For this review, take the finished solid that the model builds, in its own axes (mm). A direction names the side the tool comes from. Coordinates: 2 decimals unless noted, no trailing zeros. Loops run counter-clockwise (first coordinate to the right, second up) from the corner with the lowest first, then second, coordinate; pieces in that order, holes last. Notation, with made-up numbers: (46.25, -16) - (82.25, -16) arc R17 cw to (82.25, 2) - close; hole circle Ø7 at (66, -21). An arc over 180 degrees is marked (long way). Answer as a JSON object with one key per item and string values. Group by question number.
Item 1: Tool access review of faces 1 (the flat face through (-1.727, -0.979, 9.569)), 2 (the flat face through (0, 0, 0)): name each direction out of +Z, -Z, +X, -X, +Y, -Y from which nothing blocks a thin tool from reaching the whole face with its end or side.
Item 2: To check wall thickness, follow line 1 (Y direction, x = 0, z = 11) (3 decimals); line 2 (Z direction, x = 0.5, y = -1); line 3 (X direction, y = -2.25, z = 6.25). State the ranges of each line that lie inside material, in increasing order.
Item 3: Clearance check with flat-ended pins moving along their axes: pin 1 (2 mm diameter, centred on x = -2.5, z = 10.5, fed in from -Y); pin 2 (1.5 mm diameter, centred on y = 2.5, z = 6, fed in from +X). State where each tip first meets the part, or that it passes through.
Item 4: Mouldability with a two-part tool opening along Y and no side actions: class faces 3 (the flat face through (-1.71, 1.01, 9.57)), 4 (the cylindrical face through (3.666, 1.52, 6.269)), 5 (the flat face through (1.71, -1.01, 9.57)), 6 (the flat face through (-2, -1, 12.7)) as released by +Y, released by -Y, zero draft, split by the parting line, or undercut.
Item 5: We need section A-A (z = 8.75). Give the boundary of the cut face in (x, y) (3 decimals).
Item 6: We need section C-C (z = 3.25). Give the boundary of the cut face in (x, y).
Solid Edge part; units mm, degrees
sketch "Sketch1" plane through (0, 0, 0) normal (0, 0, 1) x (1, 0, 0)
  circle A0 centre (0, 0) radius 3.9688
extrude "Protrusion1" add sketch "Sketch1" along normal blind 12.7
chamfer "Chamfer1" distance 0.5953 angle 45 2 edges at (-3.9687, 0, 0) (-3.9687, 0, 12.7)
sketch "Sketch2" plane through (0, 0, 12.7) normal (0, 0, 1) x (1, 0, 0)
  line L0 (-1.146, 1.985) -> (1.146, 1.985)
  line L1 (2.2921, 0) -> (1.146, 1.985)
  line L2 (1.146, -1.985) -> (2.2921, 0)
  line L3 (-1.146, -1.985) -> (1.146, -1.985)
  line L4 (-2.2921, 0) -> (-1.146, -1.985)
  line L5 (-1.146, 1.985) -> (-2.2921, 0)
extrude "Cutout1" cut sketch "Sketch2" against normal blind 6.35
properties part number "24107663"
Check sheet entries:
{
 "1": {"face 1": "+Z", "face 2": "-Z, +X, -X, +Y, -Y"},
 "2": {"line 1": "y = -3.969 to -1.985, 1.985 to 3.969", "line 2": "z = 0 to 6.35", "line 3": "x = -3.27 to 3.27"},
 "3": {"pin 1": "stops at y = -3.67", "pin 2": "stops at x = 3.56"},
 "4": {"face 3": "undercut", "face 4": "split by the parting line", "face 5": "undercut", "face 6": "zero draft"},
 "5": {"outline": "circle Ø7.938 at (0, 0); hole (-2.292, 0) - (-1.146, -1.985) - (1.146, -1.985) - (2.292, 0) - (1.146, 1.985) - (-1.146, 1.985) - close"},
 "6": {"outline": "circle Ø7.94 at (0, 0)"}
}
